Check sheet for the modelled part. Datum: model origin and axes. Units: mm. Face numbers are marked on the shaded views. Round coordinates to 2 decimals unless told otherwise and drop trailing zeros. Loops run counter-clockwise (first coordinate to the right, second up) from the corner with the lowest first, then second, coordinate; pieces in that order, holes last. Notation, with made-up numbers: (27.25, 19.5) - (67.25, 19.5) arc R15 cw to (67.25, 47.5) - close; hole circle Ø1 at (-24.5, 3.5). An arc over 180 degrees is marked (long way). Put each result on its own line as item: value. Start each with the question number.
Item 1: Section check C-C, the plane x = -2. Record the cut outline in (y, z).
Item 2: Material ranges on line 1 along X through (y, z) = (-3, 60); line 2 along Y through (x, z) = (0, 3), recorded low to high.
Item 3: Section check B-B, the plane z = 167. Record the cut outline in (x, y).
Item 4: Gauge pin test, flat ends, axial feed: pin 1 Ø11.5 at (x, y) = (8, -5) entering from +Z; pin 2 Ø16.5 at (x, y) = (0, 0) entering from -Z; pin 3 Ø3.5 at (x, y) = (-2.5, -21.5) entering from -Z; pin 4 Ø1.9 at (x, z) = (1.5, 2) entering from -Y. Record the tip position at first contact, or that the pin passes through.
Item 5: Section check D-D, the plane x = -16.5. Record the cut outline in (y, z).
Item 6: Section check A-A, the plane y = 0. Record the cut outline in (x, z), and give its area (3 significant figures).
Item 7: Draft check along Y on the marked faces 1, 2 and 3. Enter one of: pulls with the +Y half, pulls with the -Y half, needs draft (parallel to the pull), parting line crosses it, or undercut.
from build123d import *

# Parameters (mm, degrees)
F0_W     = 50.8
F0_H     = 50.8
F0_W_2   = 38.1
F0_H_2   = 38.1
F1_DEPTH = 254
F2_W     = 38.1
F2_H     = 50.8
F3_DEPTH = 6.35
F4_W     = 38.1
F4_H     = 38.1
F4_R     = 6.35
F5_DEPTH = 6.35
F6_R     = 5.08


with BuildPart() as f1:
    # F0 (on Top) → F1 (new body)
    with BuildSketch(Plane.XY):
        Rectangle(F0_W, F0_H)
        Rectangle(F0_W_2, F0_H_2, mode=Mode.SUBTRACT)
    extrude(amount=F1_DEPTH)

    # F2 (on face) → F3 (cut)
    with BuildSketch(Plane.XZ.offset(25.4)):
        with Locations((0, 25.4)):
            Rectangle(F2_W, F2_H)
    extrude(amount=-F3_DEPTH, mode=Mode.SUBTRACT)

    # F4 (on Top) → F5 (join)
    with BuildSketch(Plane.XY):
        Rectangle(F4_W, F4_H)
        Circle(F4_R, mode=Mode.SUBTRACT)
    extrude(amount=F5_DEPTH)

    # F6
    f6_edges = [f1.edges().sort_by_distance(p)[0] for p in [
        (-25.4, -25.4, 127),
        (-25.4, 25.4, 127),
        (25.4, -25.4, 127),
        (25.4, 25.4, 127),
        (-19.05, 19.05, 130.175),
        (19.05, 19.05, 130.175),
        (-19.05, -19.05, 152.4),
        (19.05, -19.05, 152.4),
    ]]
    fillet(f6_edges, radius=F6_R)


solid = f1.part
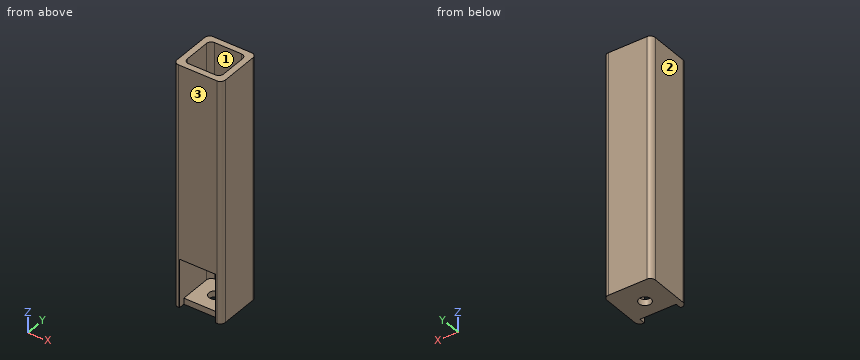
Check result:
1. outline: (-25.4, 50.8) - (-19.05, 50.8) - (-19.05, 254) - (-25.4, 254) - close; (-19.05, 0) - (-6.03, 0) - (-6.03, 6.35) - (-19.05, 6.35) - close; (6.03, 0) - (25.4, 0) - (25.4, 254) - (19.05, 254) - (19.05, 6.35) - (6.03, 6.35) - close
2. line 1: -25.4 to -19.05, 19.05 to 25.4
2. line 2: -19.05 to -6.35, 6.35 to 25.4
3. outline: (-25.4, -20.32) arc R5.08 ccw to (-20.32, -25.4) - (20.32, -25.4) arc R5.08 ccw to (25.4, -20.32) - (25.4, 20.32) arc R5.08 ccw to (20.32, 25.4) - (-20.32, 25.4) arc R5.08 ccw to (-25.4, 20.32) - close; hole (-19.05, -13.97) arc R5.08 ccw to (-13.97, -19.05) - (13.97, -19.05) arc R5.08 ccw to (19.05, -13.97) - (19.05, 13.97) arc R5.08 ccw to (13.97, 19.05) - (-13.97, 19.05) arc R5.08 ccw to (-19.05, 13.97) - close
4. pin 1: z = 6.35
4. pin 2: z = 0
4. pin 3: z = 50.8
4. pin 4: y = -19.05
5. outline: (-25.4, 50.8) - (-18.38, 50.8) - (-18.38, 254) - (-25.4, 254) - close; (-19.05, 0) - (25.4, 0) - (25.4, 254) - (18.38, 254) - (18.38, 6.35) - (-19.05, 6.35) - close
6. outline: (-25.4, 0) - (-6.35, 0) - (-6.35, 6.35) - (-19.05, 6.35) - (-19.05, 254) - (-25.4, 254) - close; (6.35, 0) - (25.4, 0) - (25.4, 254) - (19.05, 254) - (19.05, 6.35) - (6.35, 6.35) - close
6. area: 3,390 mm²
7. face 1: undercut
7. face 2: needs draft
7. face 3: pulls with the -Y half
